from build123d import *

# Parameters (mm, degrees)
F1_W        = 75
F1_H        = 90
F2_DEPTH    = 6
F3_W        = 75
F3_H        = 19
F4_DEPTH    = 23
F5_R        = 6
F6_DEPTH    = 19
F7_W        = 44
F7_H        = 16
F8_DEPTH    = 15
F9_T        = 3
F9_T3_DEPTH = 81
F9_T5_DEPTH = 22
F9_T7_DEPTH = 50
F10_R       = 4.99999
F11_W       = 20
F11_H       = 10
F12_DEPTH   = 20
F13_R       = 7.5
F14_DEPTH   = 40
F15_R       = 5


# Not quite as in the source:
# - a fillet or chamfer is up to 0.001 mm smaller than in the source, because OpenCascade refuses the exact size
# - a shell that OpenCascade refuses in one call is made with other operations: the cavity is built on its own and cut out


with BuildPart() as f2:
    # F1 (on Front) → F2 (new body)
    with BuildSketch(Plane.XZ):
        with Locations((2.5936549902, -11.7762294412)):
            Rectangle(F1_W, F1_H)
    extrude(amount=F2_DEPTH)

    # F3 (on face) → F4 (join)
    with BuildSketch(Plane.XZ.offset(6)):
        with Locations((2.5936549902, -47.2762294412)):
            Rectangle(F3_W, F3_H)
    extrude(amount=F4_DEPTH)

    # F5 (on face) → F6 (cut, through all)
    with BuildSketch(Plane.XY.offset(-37.7762294412)):
        with Locations((-26.4063450098, -17.5)):
            Circle(F5_R)
        with Locations((31.5936549902, -17.5)):
            Circle(F5_R)
    extrude(amount=-F6_DEPTH, mode=Mode.SUBTRACT)

    # F7 (on face) → F8 (join)
    with BuildSketch(Plane.XZ.offset(6)):
        with Locations((2.5936549902, 15.2237705588)):
            Rectangle(F7_W, F7_H)
    extrude(amount=F8_DEPTH)

    # F9: shell of thickness 3, made by hand


with BuildPart() as f9_core1:
    # F9_t2: copy of F2
    add(f2.part)

    # the walls: a layer under each face that stays
    f9_faces = [f9_core1.faces().sort_by_distance(p)[0] for p in [
        (40.0936549902, -24.1666666667, -41.7762294412),
        (2.5936549902, -14.5, -56.7762294412),
        (2.5936549902, -29, -47.2762294412),
        (2.5936549902, -17.5, -37.7762294412),
        (2.5936549902, -6, -2.2762294412),
        (2.5936549902, -3, 33.2237705588),
        (2.5936549902, 0, -11.7762294412),
        (-34.9063450098, -4.8333333333, 18.2237705588),
        (-32.4063450098, -17.5, -47.2762294412),
        (25.5936549902, -17.5, -47.2762294412),
        (24.5936549902, -13.5, 15.2237705588),
        (2.5936549902, -13.5, 23.2237705588),
        (-19.4063450098, -13.5, 15.2237705588),
        (2.5936549902, -13.5, 7.2237705588),
    ]]
    thicken(f9_faces, amount=-F9_T, mode=Mode.SUBTRACT)

    # F9_s4 → F9_t3 (cut)
    with BuildSketch(Plane.YZ.offset(-37.9063450098)):
        Polygon((-6.03, -37.7462294412), (-6, -40.7762294412), (-3, -40.7762294412), (-3, -37.7762294412), align=None)
    extrude(amount=F9_T3_DEPTH, mode=Mode.SUBTRACT)

    # F9_s6 → F9_t5 (cut)
    with BuildSketch(Plane.XY.offset(4.2237705588)):
        Polygon((24.6236549902, -6.03), (24.5936549902, -3), (21.5936549902, -3), (21.5936549902, -6), align=None)
        Polygon((-19.4363450098, -6.03), (-19.4063450098, -3), (-16.4063450098, -3), (-16.4063450098, -6), align=None)
    extrude(amount=F9_T5_DEPTH, mode=Mode.SUBTRACT)

    # F9_s8 → F9_t7 (cut)
    with BuildSketch(Plane.YZ.offset(-22.4063450098)):
        Polygon((-6.03, 23.2537705588), (-3, 23.2237705588), (-3, 20.2237705588), (-6, 20.2237705588), align=None)
        Polygon((-6.03, 7.1937705588), (-3, 7.2237705588), (-3, 10.2237705588), (-6, 10.2237705588), align=None)
    extrude(amount=F9_T7_DEPTH, mode=Mode.SUBTRACT)


with BuildPart() as f2_1:
    add(f2.part)

    # what is left inside the walls is the cavity
    f9_cavity = [f9_core1.part.solids().sort_by_distance(p)[0] for p in [
        (35.892563, -25.441051, -49.442896),
        (-30.705253, -25.441051, -49.442896),
        (2.593655, -18.333333, -40.806229),
        (2.593655, -15, 10.253771),
    ]]
    add(f9_cavity, mode=Mode.SUBTRACT)

    # F10 (radius 5 in the source; OpenCascade refuses exactly that, so slightly less here)
    f10_edges = [f2_1.edges().sort_by_distance(p)[0] for p in [
        (-19.406345, -13.5, 23.223771),
        (-16.406345, -13.5, 20.223771),
        (-16.406345, -13.5, 10.223771),
        (-19.406345, -13.5, 7.223771),
        (21.593655, -13.5, 20.223771),
        (21.593655, -13.5, 10.223771),
        (24.593655, -13.5, 7.223771),
        (24.593655, -13.5, 23.223771),
    ]]
    fillet(f10_edges, radius=F10_R)

    # F11 (on face) → F12 (join)
    with BuildSketch(Plane(origin=(0, 0, 0), x_dir=(-1, 0, 0), z_dir=(0, 1, 0))):
        with Locations((-2.5936549902, -11.7762294412)):
            Rectangle(F11_W, F11_H)
        with Locations((-2.5936549902, -41.7762294412)):
            Rectangle(F11_W, F11_H)
    extrude(amount=F12_DEPTH)

    # F13 (on face) → F14 (cut, through all)
    with BuildSketch(Plane.XY.offset(-6.7762294412)):
        with Locations((2.5936549902, 10)):
            Circle(F13_R)
    extrude(amount=-F14_DEPTH, mode=Mode.SUBTRACT)

    # F15
    f15_edges = [f2_1.edges().sort_by_distance(p)[0] for p in [
        (12.593655, 20, -11.776229),
        (-7.406345, 20, -11.776229),
        (-7.406345, 0, -11.776229),
        (12.593655, 0, -11.776229),
        (12.593655, 0, -41.776229),
        (12.593655, 20, -41.776229),
        (-7.406345, 0, -41.776229),
        (-7.406345, 20, -41.776229),
    ]]
    fillet(f15_edges, radius=F15_R)


solid = f2_1.part
Read the model definition and answer for the solid it produces. Units are mm, in the model's axes. A direction names the side the tool comes from. Round coordinates to 2 decimals unless told otherwise and drop trailing zeros. Order: outer loops, then holes, each group sorted by start corner. A loop starts at its lowest first (then second) coordinate and runs counter-clockwise, first axis right, second up.
1) Straight lines are drawn through the part: L1, parallel to Z at x = -4.5, y = -17.5; L2, parallel to X at y = -17, z = -46; L3, parallel to Z at x = 34.5, y = -4. For each, find the intervals that lie inside material, in ascending order.
2) The mould has two halves that part along Z. Classify faces 6 (the face through (-4, 6, -46.776)), 7 (the face through (2, -12, -53.776)), 8 (the face through (2, -29, -47)): released by +Z, released by -Z, zero draft, split by the parting line, or undercut.
3) The part is cut by section B-B on y = 10. Write down the section's boundary in (x, z).
4) The part is cut by section C-C on x = -22. Write down the section's boundary in (y, z).
5) Flat-ended cylindrical pins translate along their axes: pin 1 (6 mm diameter, centred on x = -13, y = -14, fed in from +Z); pin 2 (0.8 mm diameter, centred on x = -30, z = -48.5, fed in from +Y); pin 3 (10 mm diameter, centred on x = 1, y = 13, fed in from -Z); pin 4 (5 mm diameter, centred on x = -4, z = -43, fed in from +Y). Find the tip coordinate at first contact, or state that the pin passes through.
6) The part is cut by section A-A on y = -17.5. Give the number of separate pieces and of enclosed holes in the cut face, plus the area to 3 significant figures.
7) For faces 1 (the face through (12.594, 10, -42)), 2 (the face through (-4, 6, -36.776)), 3 (the face through (-18.39, -13.41, -47.19)), 4 (the face through (-8.91, 1.426, -41.706)), 5 (the face through (2, -12, 10.224)), determine the directions among +Z, -Z, +X, -X, +Y, -Y from which every point of the face is accessible in a straight line to the end or side of a thin tool.
8) The part is cut by section D-D on z = -14. Write down the section's boundary in (x, y).
Resolved:
1. L1: z = -56.78 to -53.78, -40.78 to -37.78, 7.22 to 10.22, 20.22 to 23.22
1. L2: x = -34.91 to -32.39, -20.43 to -17.42, 22.61 to 25.61, 37.57 to 40.09
1. L3: z = -56.78 to -53.78, -40.78 to 33.22
2. face 6: released by -Z
2. face 7: undercut
2. face 8: zero draft
3. outline: (-7.41, -46.78) - (-4.91, -46.78) - (-4.91, -36.78) - (-7.41, -36.78) - close; (-7.41, -16.78) - (-4.91, -16.78) - (-4.91, -6.78) - (-7.41, -6.78) - close; (10.09, -46.78) - (12.59, -46.78) - (12.59, -36.78) - (10.09, -36.78) - close; (10.09, -16.78) - (12.59, -16.78) - (12.59, -6.78) - (10.09, -6.78) - close
4. outline: (-29, -56.78) - (-21.57, -56.78) - (-21.57, -37.78) - (-29, -37.78) - close; (-13.43, -56.78) - (0, -56.78) - (0, 33.22) - (-6, 33.22) - (-6, -37.78) - (-13.43, -37.78) - close; hole (-26, -53.78) - (-25.35, -53.78) - (-25.35, -40.78) - (-26, -40.78) - close; hole (-9.65, -53.78) - (-3, -53.78) - (-3, -40.78) - (-9.65, -40.78) - close
5. pin 1: stops at z = 23.22
5. pin 2: stops at y = 0
5. pin 3: stops at z = -46.78
5. pin 4: stops at y = 20
6. separate pieces: 4
6. enclosed holes: 2
6. area: 773 mm2
7. face 1: +Z, -Z, +X, +Y
7. face 2: +X, -X, +Y
7. face 3: none
7. face 4: +Z, -Z, -X, +Y
7. face 5: -Y
8. outline: (-34.91, -6) - (40.09, -6) - (40.09, 0) - (17.59, 0) arc R5 cw to (12.59, 5) - (12.59, 15) arc R5 ccw to (7.59, 20) - (-2.41, 20) arc R5 ccw to (-7.41, 15) - (-7.41, 5) arc R5 cw to (-12.41, 0) - (-34.91, 0) - close; hole circle Ø15 at (2.59, 10)
